The model under review builds one solid part; all positions refer to its coordinate system, in mm. A direction names the side the tool comes from. Give positions to 0.01 mm unless a question says otherwise; leave off trailing zeros. Order: outer loops, then holes, each group sorted by start corner. A loop starts at its lowest first (then second) coordinate and runs counter-clockwise, first axis right, second up. Notation, with made-up numbers: (67.25, 18) - (75.25, 18) arc R16 ccw to (75.25, 47) - close; hole circle Ø7 at (71, -39). An arc over 180 degrees is marked (long way). Put each result on its own line as item: value.
```python
from build123d import *

# Parameters (mm, degrees)
F0_W      = 126.2948513031
F0_H      = 6.7450292408
F1_DEPTH  = 25.4
F4_R      = 2.8033052418
F5_DEPTH  = 127
F6_R      = 6.8744186216
F6_R_2    = 2.9001482236
F7_DEPTH  = 126.492
F9_DEPTH  = 12.7
F11_DEPTH = 12.7


# Not quite as in the source:
# - the program builds the solid bodies; features that only make, move or delete a surface that nothing else refers to are left out


with BuildPart() as f1:
    # F0 (on Top) → F1 (new body)
    with BuildSketch(Plane.XY):
        Rectangle(F0_W, F0_H)
    extrude(amount=F1_DEPTH)

    # F4 (on face) → F5 (cut)
    with BuildSketch(Plane(origin=(-63.1474256516, 0, 0), x_dir=(0, -1, 0), z_dir=(-1, 0, 0))):
        with Locations((-3.3725146204, 12.7)):
            Circle(F4_R)
    extrude(amount=-F5_DEPTH, mode=Mode.SUBTRACT)

    # F6 (on face) → F7 (join)
    with BuildSketch(Plane.YZ.offset(63.1474256516)):
        with Locations((3.3725146204, 12.7)):
            Circle(F6_R)
        with Locations((3.3725146204, 12.7)):
            Circle(F6_R_2, mode=Mode.SUBTRACT)
    extrude(amount=-F7_DEPTH)

    # F8 (on face) → F9 (cut)
    with BuildSketch(Plane.XZ.offset(3.3725146204)):
        Polygon((-45.5430149111, 19.8489452356), (-47.1694619385, 22.3956269569), (-50.1881765182, 22.2604233738), (-51.5804440704, 19.5785380695), (-49.953997043, 17.0318563483), (-46.9352824633, 17.1670599313), align=None)
    extrude(amount=-F9_DEPTH, mode=Mode.SUBTRACT)

    # F10 (on face) → F11 (cut)
    with BuildSketch(Plane.XZ.offset(3.3725146204)):
        Polygon((5.2098441705, 19.6924402974), (3.583397143, 22.2391220187), (0.5646825633, 22.1039184357), (-0.8275849889, 19.4220331314), (0.7988620385, 16.8753514101), (3.8175766182, 17.0105549931), align=None)
    extrude(amount=-F11_DEPTH, mode=Mode.SUBTRACT)


solid = f1.part
```
(1) Take a section at D-D, the plane z = 3.25. Write out the cut boundary in (x, y).
The answers:
outline: (-63.15, -3.37) - (63.15, -3.37) - (63.15, 3.37) - (-63.15, 3.37) - close
(2) For faces 5 (the flat face through (-63.147, 0, 3)), 6 (the flat face through (-63.147, 0, 22)), 7 (the flat face through (-48.66, -0.05, 22.33)), 8 (the flat face through (-1, -3.373, 20)), 9 (the flat face through (-1, 3.373, 3)), list the 3-axis set-ups (+Z, -Z, +X, -X, +Y, -Y) from which the entire face can be reached by the end or side of a thin tool; tool diameter is ignored.
The answers:
face 5: -Z, -X, -Y
face 6: +Z, -X, -Y
face 7: +Y, -Y
face 8: +Z, +X, -X, -Y
face 9: -Z, +X, -X, +Y
(3) Clearance check with flat-ended pins moving along their axes: pin 1 Ø6 at (x, z) = (1, 6) entering from -Y; pin 2 Ø2 at (x, y) = (5, 5.5) entering from -Z; pin 3 Ø3 at (y, z) = (3.5, 22.5) entering from -X; pin 4 Ø12 at (x, z) = (-33.5, 18.5) entering from -Y. State where each tip first meets the part, or that it passes through.
The answers:
pin 1: y = -3.37
pin 2: z = 5.92
pin 3: x = -63.15
pin 4: y = -3.5
(4) Take a section at C-C, the plane x = 34. Write out the cut boundary in (y, z), then the cut area to 3 significant figures.
The answers:
outline: (-3.37, 0) - (3.37, 0) - (3.37, 5.83) arc R6.87 ccw to (3.37, 19.57) - (3.37, 25.4) - (-3.37, 25.4) - (-3.37, 14.03) arc R6.87 ccw to (-3.37, 11.37) - close; hole (3.37, 9.8) arc R2.9 ccw to (3.37, 15.6) - (3.37, 15.5) arc R2.8 ccw to (3.37, 9.9) - close
area: 220 mm^2
(5) Wall thickness on L1, parallel to Y at x = 16, z = 12.7; L2, parallel to Z at x = -47, y = 1; L3, parallel to Z at x = -46, y = 6: over which ranges is each line inside the solid? List them lowest first.
The answers:
L1: -3.5 to 0.57, 6.27 to 10.25
L2: 0 to 11.21, 14.19 to 17.16, 22.13 to 25.4
L3: 6.35 to 11.47, 13.93 to 18.97
(6) Take a section at A-A, the plane z = 12.7. Write out the cut boundary in (x, y), then the cut area to 3 significant figures.
The answers:
outline: (-63.34, -3.5) - (63.15, -3.5) - (63.15, 0.57) - (-63.15, 0.57) - (-63.15, 0.47) - (-63.34, 0.47) - close; (-63.34, 6.27) - (63.15, 6.27) - (63.15, 10.25) - (-63.34, 10.25) - close
area: 1,020 mm^2
(7) Take a section at B-B, the plane y = 2. Write out the cut boundary in (x, z).
The answers:
outline: (-63.34, 5.96) - (-63.15, 5.96) - (-63.15, 0) - (63.15, 0) - (63.15, 10.26) - (-63.15, 10.26) - (-63.15, 10.15) - (-63.34, 10.15) - close; (-63.34, 15.25) - (-63.15, 15.25) - (-63.15, 15.14) - (63.15, 15.14) - (63.15, 25.4) - (-63.15, 25.4) - (-63.15, 19.44) - (-63.34, 19.44) - close; hole (-51.58, 19.58) - (-49.95, 17.03) - (-46.94, 17.17) - (-45.54, 19.85) - (-47.17, 22.4) - (-50.19, 22.26) - close; hole (-0.83, 19.42) - (0.8, 16.88) - (3.82, 17.01) - (5.21, 19.69) - (3.58, 22.24) - (0.56, 22.1) - close
(8) The part is to be moulded in two halves that separate along Y. For faces 1 (the cylindrical face through (0.79, 6.14, 13.57)), 2 (the cylindrical face through (0.787, 9.723, 10.067)), 3 (the flat face through (-46.25, 1.2, 18.49)), 4 (the flat face through (-1, 3.373, 22)), say which applies: pulls with the +Y half, pulls with the -Y half, needs draft (parallel to the pull), parting line crosses it, or undercut.
The answers:
face 1: undercut
face 2: parting line crosses it
face 3: needs draft
face 4: pulls with the +Y half
